from build123d import *

# Parameters (mm, degrees)
SKETCH_1_W          = 35.5
SKETCH_1_H          = 37.5
EXTRUDE_1_DEPTH     = 30
SKETCH_2_W          = 41.5
SKETCH_2_H          = 43.5
EXTRUDE_2_DEPTH     = 3
SKETCH_4_W          = 5.142655321
SKETCH_4_H          = 10.097164716
SKETCH_4_W_2        = 5.20537063
SKETCH_4_H_2        = 11.037894348
CUT_EXTRUDE_1_DEPTH = 25


with BuildPart() as part:
    # 草图1 → 凸台-拉伸1 (new body)
    with BuildSketch(Plane(origin=(0, 0, 0), x_dir=(1, 0, 0), z_dir=(0, 1, 0))):
        Rectangle(SKETCH_1_W, SKETCH_1_H)
    extrude(amount=EXTRUDE_1_DEPTH)

    # 草图2 → 凸台-拉伸2 (add)
    with BuildSketch(Plane(origin=(0, 30, 0), x_dir=(1, 0, 0), z_dir=(0, 1, 0))):
        Rectangle(SKETCH_2_W, SKETCH_2_H)
    extrude(amount=EXTRUDE_2_DEPTH)

    # 草图4 → 切除-拉伸1 (cut)
    with BuildSketch(Plane(origin=(0, 33, 0), x_dir=(1, 0, 0), z_dir=(0, 1, 0))):
        with Locations((11.02137602, -10.787033113)):
            Rectangle(SKETCH_4_W, SKETCH_4_H)
        with Locations((-0.344934198, 8.686070268)):
            Rectangle(SKETCH_4_W_2, SKETCH_4_H_2)
        with Locations((-11.97862398, -10.787033113)):
            Rectangle(SKETCH_4_W, SKETCH_4_H)
    extrude(amount=-CUT_EXTRUDE_1_DEPTH, mode=Mode.SUBTRACT)


solid = part.part
Read the model definition and answer for the solid it produces. Units are mm, in the model's axes. A direction names the side the tool comes from. Give positions to 0.01 mm unless a question says otherwise; leave off trailing zeros. Loops run counter-clockwise (first coordinate to the right, second up) from the corner with the lowest first, then second, coordinate; pieces in that order, holes last. Notation, with made-up numbers: (53, 23) -> (64, 23) arc R23 cw to (64, 37) -> close; hole circle Ø5 at (37, 32.25). An arc over 180 degrees is marked (long way). Use a Markdown table: item, result.
Q1. Section A-A, the plane y = 17 is taken. Determine the outline of the cut face in (x, z).
Solved:
| item | result |
|---|---|
| outline | (-17.75, -18.75) -> (17.75, -18.75) -> (17.75, 18.75) -> (-17.75, 18.75) -> close; hole (-14.55, 5.74) -> (-9.41, 5.74) -> (-9.41, 15.84) -> (-14.55, 15.84) -> close; hole (-2.95, -14.21) -> (2.26, -14.21) -> (2.26, -3.17) -> (-2.95, -3.17) -> close; hole (8.45, 5.74) -> (13.59, 5.74) -> (13.59, 15.84) -> (8.45, 15.84) -> close |
Q2. Section C-C, the plane x = -8 is taken. Determine the outline of the cut face in (y, z).
Solved:
| item | result |
|---|---|
| outline | (0, -18.75) -> (30, -18.75) -> (30, -21.75) -> (33, -21.75) -> (33, 21.75) -> (30, 21.75) -> (30, 18.75) -> (0, 18.75) -> close |
Q3. A tool of negligible diameter and unlimited length cuts with its end or side. For faces 1 (the face through (0, 31, 21.75)), 2 (the face through (8.45, 21, 11)), 3 (the face through (0, 15, -18.75)), from which of +Z, -Z, +X, -X, +Y, -Y can it reach the whole face along a straight path? Write none if from no direction.
Solved:
| item | result |
|---|---|
| face 1 | +Z, +X, -X, +Y, -Y |
| face 2 | +Y |
| face 3 | -Z, +X, -X, -Y |
Q4. Each of these flat-tipped pins is pushed along its axis until it touches: pin 1 (2 mm diameter, centred on x = -6, y = 16, fed in from -Z); pin 2 (1 mm diameter, centred on x = 7.5, y = 16, fed in from +Z); pin 3 (2 mm diameter, centred on y = 9, z = 4.5, fed in from +X); pin 4 (10 mm diameter, centred on x = 14, z = -6, fed in from -Y). Where does it stop, or does it pass through?
Solved:
| item | result |
|---|---|
| pin 1 | stops at z = -18.75 |
| pin 2 | stops at z = 18.75 |
| pin 3 | stops at x = 17.75 |
| pin 4 | stops at y = 0 |
Q5. Determine the mould class of faces 4 (the face through (0, 21, -14.205)), 5 (the face through (-14.55, 21, 11)), 6 (the face through (17.75, 15, 0)), 7 (the face through (0, 15, 18.75)) for opening direction X: pulls with the +X half, pulls with the -X half, needs draft (parallel to the pull), parting line crosses it, or undercut.
Solved:
| item | result |
|---|---|
| face 4 | undercut |
| face 5 | undercut |
| face 6 | pulls with the +X half |
| face 7 | needs draft |
Q6. Find the intervals of material crossed by line 1 along X through (y, z) = (18, 6); line 2 along X through (y, z) = (21, -4); line 3 along Z through (x, y) = (13, 26), in increasing order.
Solved:
| item | result |
|---|---|
| line 1 | x = -17.75 to -14.55, -9.41 to 8.45, 13.59 to 17.75 |
| line 2 | x = -17.75 to -2.95, 2.26 to 17.75 |
| line 3 | z = -18.75 to 5.74, 15.84 to 18.75 |
Q7. Section D-D, the plane z = -16.5 is taken. Determine the outline of the cut face in (x, y), then the cut area to 3 significant figures.
Solved:
| item | result |
|---|---|
| outline | (-20.75, 30) -> (-17.75, 30) -> (-17.75, 0) -> (17.75, 0) -> (17.75, 30) -> (20.75, 30) -> (20.75, 33) -> (-20.75, 33) -> close |
| area | 1,190 mm^2 |
Q8. Section B-B, the plane z = 12.5 is taken. Determine the outline of the cut face in (x, y), then the cut area to 3 significant figures.
Solved:
| item | result |
|---|---|
| outline | (-20.75, 30) -> (-17.75, 30) -> (-17.75, 0) -> (17.75, 0) -> (17.75, 30) -> (20.75, 30) -> (20.75, 33) -> (13.59, 33) -> (13.59, 8) -> (8.45, 8) -> (8.45, 33) -> (-9.41, 33) -> (-9.41, 8) -> (-14.55, 8) -> (-14.55, 33) -> (-20.75, 33) -> close |
| area | 932 mm^2 |
